Could you check a few things on this drawing? It's one solid part, dimensions in mm from its lowest x, y, z. A direction names the side the tool comes from. Give positions to 0.01 mm unless a question says otherwise; leave off trailing zeros. Order: outer loops, then holes, each group sorted by start corner. A loop starts at its lowest first (then second) coordinate and runs counter-clockwise, first axis right, second up. Notation, with made-up numbers: (-24.5, 85.25) - (26.5, 85.25) arc R31 cw to (26.5, 119.25) - close; hole circle Ø2 at (-16.75, 3.5). An arc over 180 degrees is marked (long way). Put each result on its own line as item: value.
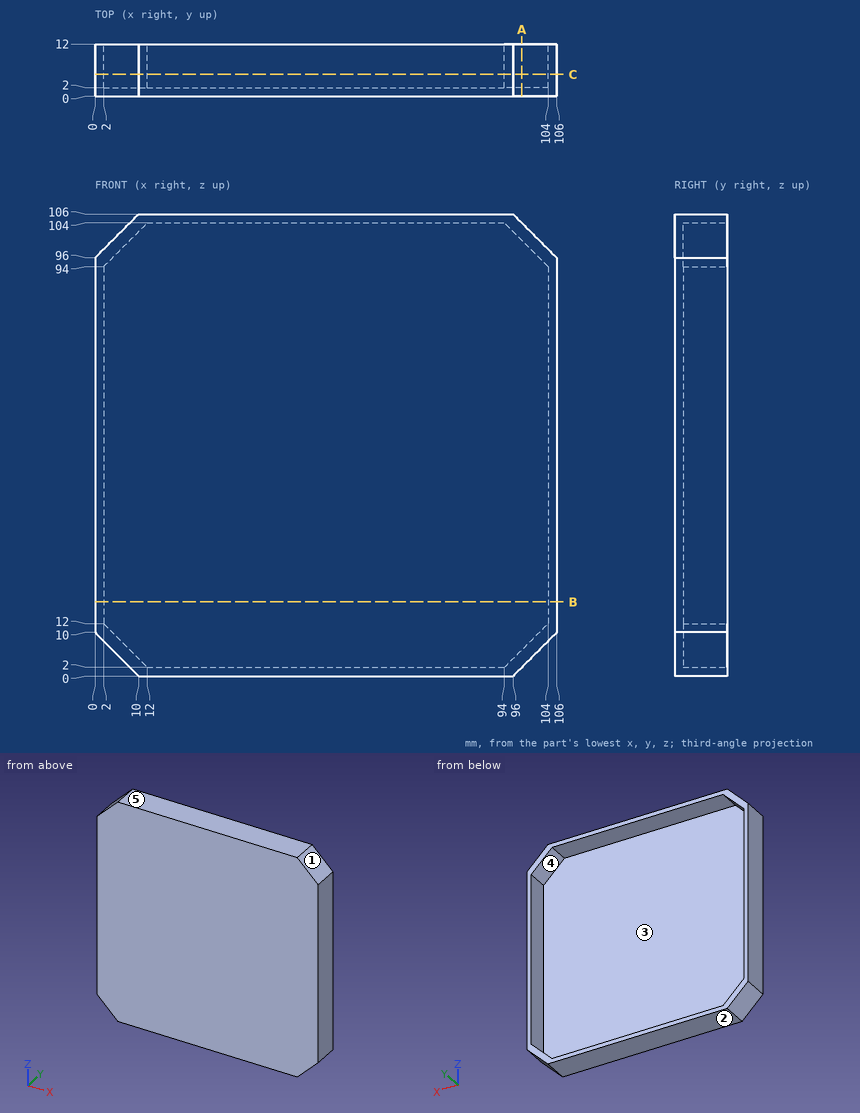
1) I'm going to push a flat-ended pin straight in: pin 1 (1.5 mm diameter, centred on x = 44.5, z = 72.5, fed in from +Y). Where does the tip first touch, or does it pass through?
Filled in:
pin 1: stops at y = 2
2) Which directions (+Z, -Z, +X, -X, +Y, -Y) give clear straight access to the entire face, cutting with the end or side of a thin tool? Please do the marked faces 4 and 5.
Filled in:
face 4: +Y
face 5: +Z, +X, -X, +Y, -Y
3) Suppose I cut it at C-C, the plane y = 5. List the corners of the cut face in (x, z) for me, and give its area (3 significant figures).
Filled in:
outline: (0, 10) - (10, 0) - (96, 0) - (106, 10) - (106, 96) - (96, 106) - (10, 106) - (0, 96) - close; hole (2, 12) - (12, 2) - (94, 2) - (104, 12) - (104, 94) - (94, 104) - (12, 104) - (2, 94) - close
area: 832 mm^2
4) Suppose I cut it at A-A, the plane x = 98. List the corners of the cut face in (y, z) for me.
Filled in:
outline: (0, 2) - (12, 2) - (12, 6) - (2, 6) - (2, 100) - (12, 100) - (12, 104) - (0, 104) - close
5) Suppose I cut it at B-B, the plane z = 17. List the corners of the cut face in (x, y) for me.
Filled in:
outline: (0, 0) - (106, 0) - (106, 12) - (104, 12) - (104, 2) - (2, 2) - (2, 12) - (0, 12) - close
6) If I drill on line 1 (X direction, y = 7.75, z = 22.5); line 2 (Y direction, x = 55, z = 88.5), over which ranges is the centre line in solid material (lowest first)? Write a range as [from, to].
Filled in:
line 1: x = [0, 2], [104, 106]
line 2: y = [0, 2]
7) We'd pull the mould along X, two halves only. Please class the marked faces 1, 2 and 3: pulls with the +X half, pulls with the -X half, needs draft (parallel to the pull), parting line crosses it, or undercut.
Filled in:
face 1: pulls with the +X half
face 2: needs draft
face 3: undercut
